```python
from build123d import *

# Parameters (mm, degrees)
F0_W      = 26
F0_H      = 26
F1_DEPTH  = 10
F2_R      = 7.5
F3_DEPTH  = 19
F5_DEPTH  = 1
F7_DEPTH  = 1
F8_R      = 1.6
F9_DEPTH  = 1
F10_R     = 1.6
F11_DEPTH = 1


with BuildPart() as f1:
    # F0 (on Front) → F1 (new body)
    with BuildSketch(Plane.XZ):
        Rectangle(F0_W, F0_H)
    extrude(amount=F1_DEPTH)

    # F2 (on face) → F3 (join)
    with BuildSketch(Plane.XZ.offset(10)):
        Circle(F2_R)
    extrude(amount=F3_DEPTH)

    # F4 (on face) → F5 (join)
    with BuildSketch(Plane.YZ.offset(13)):
        with BuildLine():
            ThreePointArc((-2.75, 0), (-5, 2.25), (-7.25, 0))
            Line((-7.25, 0), (-2.75, 0))
        make_face()
        with BuildLine():
            Line((-2.75, 0), (-7.25, 0))
            ThreePointArc((-7.25, 0), (-5, -2.25), (-2.75, 0))
        make_face()
    extrude(amount=F5_DEPTH)

    # F6 (on face) → F7 (join)
    with BuildSketch(Plane(origin=(-13, 0, 0), x_dir=(0, -1, 0), z_dir=(-1, 0, 0))):
        with BuildLine():
            ThreePointArc((7.25, 0), (5, 2.25), (2.75, 0))
            Line((2.75, 0), (7.25, 0))
        make_face()
        with BuildLine():
            Line((7.25, 0), (2.75, 0))
            ThreePointArc((2.75, 0), (5, -2.25), (7.25, 0))
        make_face()
    extrude(amount=F7_DEPTH)

    # F8 (on face) → F9 (join)
    with BuildSketch(Plane(origin=(-14, 0, 0), x_dir=(0, -1, 0), z_dir=(-1, 0, 0))):
        with Locations((5, 0)):
            Circle(F8_R)
    extrude(amount=F9_DEPTH)

    # F10 (on face) → F11 (join)
    with BuildSketch(Plane.YZ.offset(14)):
        with Locations((-5, 0)):
            Circle(F10_R)
    extrude(amount=F11_DEPTH)


solid = f1.part
```
The model under review builds one solid part; all positions refer to its coordinate system, in mm. A direction names the side the tool comes from. Round coordinates to 2 decimals unless told otherwise and drop trailing zeros. Order: outer loops, then holes, each group sorted by start corner. A loop starts at its lowest first (then second) coordinate and runs counter-clockwise, first axis right, second up.
Item 1: Add section A-A, the plane x = 0. State the section outline as (y, z) points.
Working result:
outline: (-29, -7.5) - (-10, -7.5) - (-10, -13) - (0, -13) - (0, 13) - (-10, 13) - (-10, 7.5) - (-29, 7.5) - close
Item 2: For pin 1 (6 mm diameter, centred on y = -21.5, z = 1.5, fed in from +X); pin 2 (5 mm diameter, centred on x = 2.5, y = -20, fed in from -Z); pin 3 (2 mm diameter, centred on y = -14, z = -7.5, fed in from -X), all flat-tipped, find the tip position at first contact; note any pin that passes through.
Working result:
pin 1: stops at x = 7.5
pin 2: stops at z = -7.5
pin 3: stops at x = -3.74
Item 3: Add section B-B, the plane y = -5. State the section outline as (x, z) points, and give its area (3 significant figures).
Working result:
outline: (-15, -1.6) - (-14, -1.6) - (-14, -2.25) - (-13, -2.25) - (-13, -13) - (13, -13) - (13, -2.25) - (14, -2.25) - (14, -1.6) - (15, -1.6) - (15, 1.6) - (14, 1.6) - (14, 2.25) - (13, 2.25) - (13, 13) - (-13, 13) - (-13, 2.25) - (-14, 2.25) - (-14, 1.6) - (-15, 1.6) - close
area: 691 mm2
Item 4: Add section C-C, the plane z = 0. State the section outline as (x, y) points, and give its area (3 significant figures).
Working result:
outline: (-15, -6.6) - (-14, -6.6) - (-14, -7.25) - (-13, -7.25) - (-13, -10) - (-7.5, -10) - (-7.5, -29) - (7.5, -29) - (7.5, -10) - (13, -10) - (13, -7.25) - (14, -7.25) - (14, -6.6) - (15, -6.6) - (15, -3.4) - (14, -3.4) - (14, -2.75) - (13, -2.75) - (13, 0) - (-13, 0) - (-13, -2.75) - (-14, -2.75) - (-14, -3.4) - (-15, -3.4) - close
area: 560 mm2
Item 5: Machinability: for faces 1 (the cylindrical face through (14.49, -6.6, 0.07)), 2 (the flat face through (-14, -5, 2)), 3 (the cylindrical face through (-7.493, -19.367, 0.33)), which of the approach directions +Z, -Z, +X, -X, +Y, -Y give a long, thin tool a straight path to every point of the face, cutting with its end or side? Answer none if there is none.
Working result:
face 1: +X
face 2: -X
face 3: -Y
Item 6: To check wall thickness, follow probe 1 along X at (y, z) = (-7.75, -2.5); probe 2 along Y at (x, z) = (-6, 7.75); probe 3 along X at (y, z) = (-19.75, 2.5). State the ranges of each line that lie inside material, in increasing order.
Working result:
probe 1: x = -13 to 13
probe 2: y = -10 to 0
probe 3: x = -7.07 to 7.07
Item 7: Add section D-D, the plane z = -5.5. State the section outline as (x, y) points, and give its area (3 significant figures).
Working result:
outline: (-13, -10) - (-5.1, -10) - (-5.1, -29) - (5.1, -29) - (5.1, -10) - (13, -10) - (13, 0) - (-13, 0) - close
area: 454 mm2
